Study the drawing (mm; zero at the part's minimum x, y, z) and answer. Round coordinates to 2 decimals unless told otherwise and drop trailing zeros. Write each question's results on one line, items separated by ' | '.
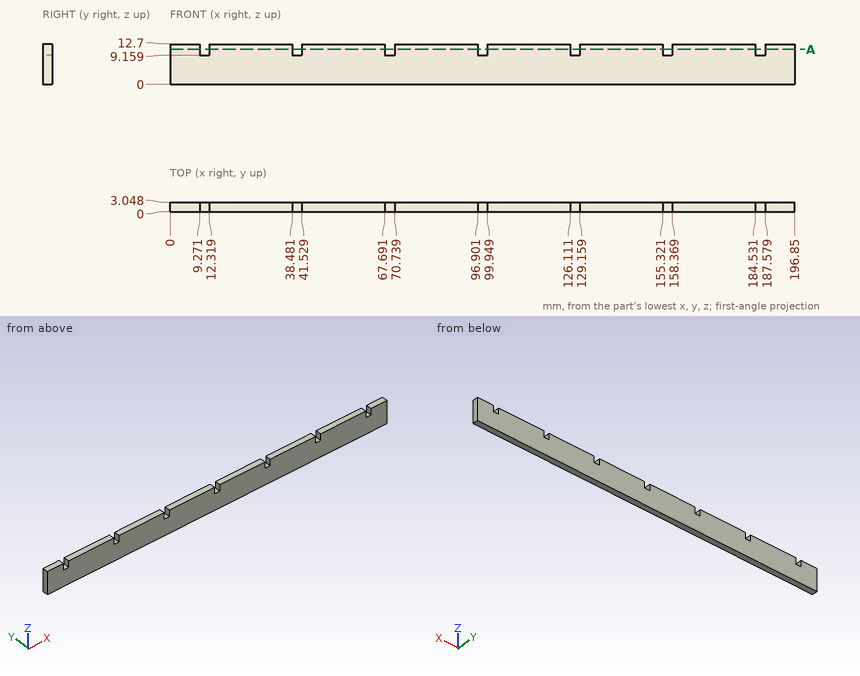
Item 1: A flat-ended cylindrical pin translates along its axis: pin 1 (1.5 mm diameter, centred on x = 10.5, y = 2, fed in from +Z). Find the tip coordinate at first contact, or state that the pin passes through.
Outcome:
pin 1: stops at z = 9.16
Item 2: The part is cut by section A-A (z = 11). State how many separate pieces and enclosed holes the cut face has, plus the area to 3 significant figures.
Outcome:
separate pieces: 8 | enclosed holes: 0 | area: 535 mm2
Item 3: A straight line is drawn through the part: line 1 (Z direction, x = 99, y = 1.1). Find the intervals that lie inside material, in ascending order.
Outcome:
line 1: z = 0 to 9.16
